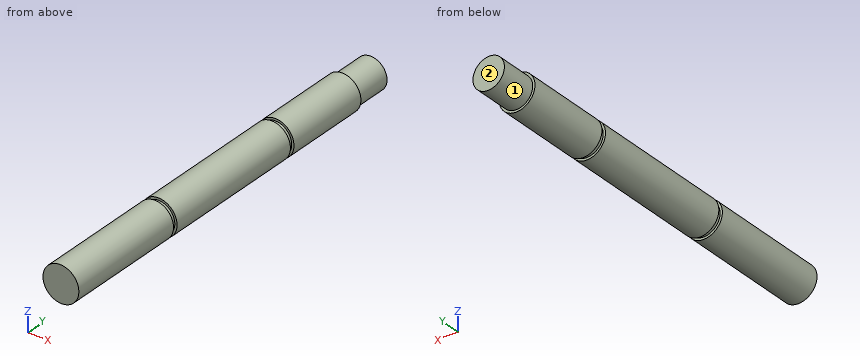
```python
from build123d import *

# Parameters (mm, degrees)
F0_R      = 6.35
F1_DEPTH  = 42.418
F2_R      = 5.55625
F3_DEPTH  = 1.5875
F4_R      = 6.35
F5_DEPTH  = 50.8
F6_R      = 5.55625
F7_DEPTH  = 1.5875
F8_R      = 6.35
F9_DEPTH  = 30.0101
F10_R     = 5.55625
F11_DEPTH = 12.7


with BuildPart() as f1:
    # F0 (on Front) → F1 (new body)
    with BuildSketch(Plane.XZ):
        Circle(F0_R)
    extrude(amount=F1_DEPTH)

    # F2 (on face) → F3 (join)
    with BuildSketch(Plane(origin=(0, 0, 0), x_dir=(-1, 0, 0), z_dir=(0, 1, 0))):
        Circle(F2_R)
    extrude(amount=F3_DEPTH)

    # F4 (on face) → F5 (join)
    with BuildSketch(Plane(origin=(0, 1.5875, 0), x_dir=(-1, 0, 0), z_dir=(0, 1, 0))):
        Circle(F4_R)
    extrude(amount=F5_DEPTH)

    # F6 (on face) → F7 (join)
    with BuildSketch(Plane(origin=(0, 52.3875, 0), x_dir=(-1, 0, 0), z_dir=(0, 1, 0))):
        Circle(F6_R)
    extrude(amount=F7_DEPTH)

    # F8 (on face) → F9 (join)
    with BuildSketch(Plane(origin=(0, 53.975, 0), x_dir=(-1, 0, 0), z_dir=(0, 1, 0))):
        Circle(F8_R)
    extrude(amount=F9_DEPTH)

    # F10 (on face) → F11 (join)
    with BuildSketch(Plane(origin=(0, 83.9851, 0), x_dir=(-1, 0, 0), z_dir=(0, 1, 0))):
        Circle(F10_R)
    extrude(amount=F11_DEPTH)


solid = f1.part
```
The listing builds one solid part. Answer for the finished solid, in the listing's coordinates (mm). Face numbers are marked on the shaded views. A direction names the side the tool comes from. Give positions to 0.01 mm unless a question says otherwise; leave off trailing zeros. Order: outer loops, then holes, each group sorted by start corner. A loop starts at its lowest first (then second) coordinate and runs counter-clockwise, first axis right, second up. Notation, with made-up numbers: (-23, -18.5) - (-10, -18.5) arc R34 cw to (-10, 11.5) - close; hole circle Ø1 at (71.25, 15.5). An arc over 180 degrees is marked (long way). Answer in a Markdown table with one row per item. Add a question column.
Q1. Given P1, Ø5, axis at y = 31, z = 3.5, coming from the +X side; P2, Ø1, axis at y = 48.5, z = -4.5, coming from the -X side; P3, Ø2, axis at y = 44, z = 5, coming from the +X side, each flat-ended and moving along its own axis, determine where each tip first touches the part or whether it passes through.
Q2. The part is cut by section A-A (x = 2.5). Determine the outline of the cut face in (y, z) (1 decimal).
Q3. Find the intervals of material crossed by line 1 along Y through (x, z) = (5.5, 1.25) (1 decimal); line 2 along Z through (x, y) = (-2.5, 33); line 3 along Z through (x, y) = (2, 75.5), in increasing order. Write a range as [from, to].
Q4. Which of the six approach directions +Z, -Z, +X, -X, +Y, -Y give full straight-line access (tool end or side, diameter ignored) to the marked faces 1 and 2?
Q5. The part is cut by section B-B (y = -21). Determine the outline of the cut face in (x, z).
Determined:
| question | item | result |
|---|---|---|
| 1 | P1 | stops at x = 6.27 |
| 1 | P2 | stops at x = -4.93 |
| 1 | P3 | stops at x = 4.93 |
| 2 | outline | (-42.4, -5.8) - (0, -5.8) - (0, -5) - (1.6, -5) - (1.6, -5.8) - (52.4, -5.8) - (52.4, -5) - (54, -5) - (54, -5.8) - (84, -5.8) - (84, -5) - (96.7, -5) - (96.7, 5) - (84, 5) - (84, 5.8) - (54, 5.8) - (54, 5) - (52.4, 5) - (52.4, 5.8) - (1.6, 5.8) - (1.6, 5) - (0, 5) - (0, 5.8) - (-42.4, 5.8) - close |
| 3 | line 1 | y = [-42.4, 0], [1.6, 52.4], [54, 84] |
| 3 | line 2 | z = [-5.84, 5.84] |
| 3 | line 3 | z = [-6.03, 6.03] |
| 4 | face 1 | +Y |
| 4 | face 2 | +Z, -Z, +X, -X, +Y |
| 5 | outline | circle Ø12.7 at (0, 0) |
